Here's the drawing with two shaded views (mm, measured from the low corner). I have some questions. Coordinates: 2 decimals unless noted, no trailing zeros. Write each loop counter-clockwise with the first axis right and the second up, starting at its lowest first coordinate (ties: lowest second). Pieces come first, ordered by that corner, then holes.
Item 1: I want a section at B-B on x = 39. Please give me the cut outline in (y, z).
Item 2: If I drill on probe 1 along Y at (x, z) = (15, 2); probe 2 along Y at (x, z) = (41, 0.6); probe 3 along X at (y, z) = (101.5, 0.9), over which ranges is the centre line in solid material (lowest first)?
Item 3: I want a section at D-D on z = 1.3. Please give me the cut outline in (x, y).
Item 4: For P1, Ø1, axis at y = 101.5, z = 2.5, coming from the +X side; P2, Ø1, axis at y = 105.5, z = 1.5, coming from the -X side; P3, Ø1, axis at y = 46, z = 2, coming from the +X side; P4, Ø6, axis at x = 35.5, y = 32.5, coming from the -Z side, each with a flat end and sliding along its axis, tell me the tip position at first contact or that it passes through.
Item 5: I want a section at A-A on y = 103.5. Please give me the cut outline in (x, z), then the cut area to 3 significant figures.
Item 6: I want a section at C-C on y = 10.5. Please give me the cut outline in (x, z).
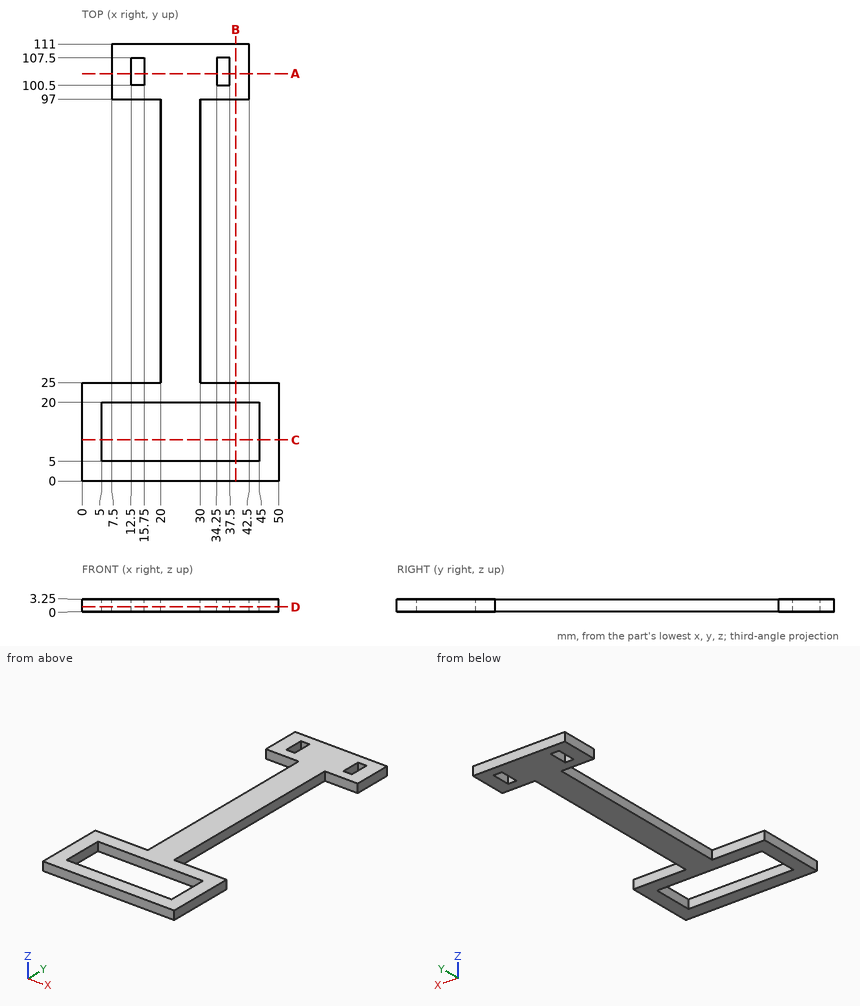
Response values:
1. outline: (0, 0) - (5, 0) - (5, 3.25) - (0, 3.25) - close; (20, 0) - (25, 0) - (25, 3.25) - (20, 3.25) - close; (97, 0) - (111, 0) - (111, 3.25) - (97, 3.25) - close
2. probe 1: y = 0 to 5, 20 to 25, 97 to 100.5, 107.5 to 111
2. probe 2: y = 0 to 5, 20 to 25, 97 to 111
2. probe 3: x = 7.5 to 12.5, 15.75 to 34.25, 37.5 to 42.5
3. outline: (0, 0) - (50, 0) - (50, 25) - (30, 25) - (30, 97) - (42.5, 97) - (42.5, 111) - (7.5, 111) - (7.5, 97) - (20, 97) - (20, 25) - (0, 25) - close; hole (5, 5) - (45, 5) - (45, 20) - (5, 20) - close; hole (12.5, 100.5) - (15.75, 100.5) - (15.75, 107.5) - (12.5, 107.5) - close; hole (34.25, 100.5) - (37.5, 100.5) - (37.5, 107.5) - (34.25, 107.5) - close
4. P1: stops at x = 42.5
4. P2: stops at x = 7.5
4. P3: stops at x = 30
4. P4: passes through
5. outline: (7.5, 0) - (12.5, 0) - (12.5, 3.25) - (7.5, 3.25) - close; (15.75, 0) - (34.25, 0) - (34.25, 3.25) - (15.75, 3.25) - close; (37.5, 0) - (42.5, 0) - (42.5, 3.25) - (37.5, 3.25) - close
5. area: 92.6 mm2
6. outline: (0, 0) - (5, 0) - (5, 3.25) - (0, 3.25) - close; (45, 0) - (50, 0) - (50, 3.25) - (45, 3.25) - close
